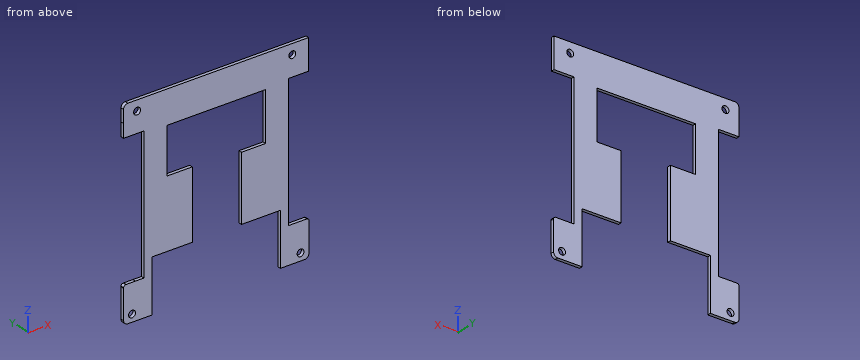
from build123d import *

# Parameters (mm, degrees)
SKETCH1_2_R                 = 1.6383
BOSS_EXTRUDE2_DEPTH         = 1.575
SKETCH2_W                   = 14.080651801
SKETCH2_H                   = 7.11628052
SKETCH2_W_2                 = 15.007196354
SKETCH2_H_2                 = 9.421332762
CUT_EXTRUDE1_DEPTH          = 65.400942629
ADDITIONAL_PCB_MATERIAL_W   = 2.649520344
ADDITIONAL_PCB_MATERIAL_H   = 65.213315835
ADDITIONAL_PCB_MATERIAL_W_2 = 1.5
ADDITIONAL_PCB_MATERIAL_H_2 = 65.299191064
BOSS_EXTRUDE3_DEPTH         = 1.575


with BuildPart() as part:
    # Sketch1_2 → Boss-Extrude2 (new body)
    with BuildSketch(Plane(origin=(0, 0, 0), x_dir=(1, 0, 0), z_dir=(0, 1, 0))):
        with BuildLine():
            Line((-38.39500299, 29.999999735), (-42.73000299, 29.999999735))
            Line((-42.73000299, 29.999999735), (-43.011025994, 30.003097626))
            ThreePointArc((-43.011025994, 30.003097626), (-43.710996344, 30.299838092), (-44.000003042, 31.003036872))
            Line((-44.000003042, 31.003036872), (-44.000003042, 31.269999735))
            Line((-44.000003042, 31.269999735), (-44.000005679, 44.999999735))
            ThreePointArc((-44.000005679, 44.999999735), (-43.414218633, 46.414215608), (-42.000002924, 47.000003051))
            Line((-42.000002924, 47.000003051), (-30.435003, 47.000003051))
            Line((-30.435003, 47.000003051), (-30.435003, 22.255357341))
            Line((-30.435003, 22.255357341), (-11.409003, 22.255357341))
            Line((-11.409003, 22.255357341), (-11.409003, -9.899999999))
            Line((-11.409003, -9.899999999), (-23.409003, -9.899999999))
            Line((-23.409003, -9.899999999), (-23.409003, -31.499996949))
            Line((-23.409003, -31.499996949), (23.408997, -31.499996949))
            Line((23.408997, -31.499996949), (23.408997, -8.499997555))
            Line((23.408997, -8.499997555), (11.97084713, -8.499997555))
            Line((11.97084713, -8.499997555), (11.97084713, 22.255357341))
            Line((11.97084713, 22.255357341), (30.434997, 22.255357341))
            Line((30.434997, 22.255357341), (30.434997, 47.000003051))
            Line((30.434997, 47.000003051), (42.000008541, 47.000003051))
            ThreePointArc((42.000008541, 47.000003051), (43.414213215, 46.414220704), (43.999996956, 45.000016607))
            Line((43.999996956, 45.000016607), (43.999996956, 32.000003378))
            Line((43.999996956, 32.000003378), (43.999996956, 31.015615364))
            ThreePointArc((43.999996956, 31.015615364), (43.706534093, 30.307939396), (42.998386406, 30.015616661))
            Line((42.998386406, 30.015616661), (33.825607551, 30.030389905))
            ThreePointArc((33.825607551, 30.030389905), (33.117459864, 29.738067169), (32.823997, 29.030391202))
            Line((32.823997, 29.030391202), (32.823997, -30.453996949))
            ThreePointArc((32.823997, -30.453996949), (33.116890219, -31.16110373), (33.823997, -31.453996949))
            Line((33.823997, -31.453996949), (36.099999555, -31.453996949))
            Line((36.099999555, -31.453996949), (42.849728118, -31.453996949))
            ThreePointArc((42.849728118, -31.453996949), (43.556834899, -31.746890168), (43.849728118, -32.453996949))
            Line((43.849728118, -32.453996949), (43.849728118, -36.999996949))
            Line((43.849728118, -36.999996949), (43.849728118, -46.999996949))
            Line((43.849728118, -46.999996949), (-42.000000178, -46.999996949))
            ThreePointArc((-42.000000178, -46.999996949), (-43.414212804, -46.414211581), (-44.000000499, -44.999999921))
            Line((-44.000000499, -44.999999921), (-44.000000178, -38.976999921))
            Line((-44.000000178, -38.976999921), (-44.000000178, -32.453999802))
            ThreePointArc((-44.000000178, -32.453999802), (-43.70710696, -31.746893021), (-43.000000178, -31.453999802))
            Line((-43.000000178, -31.453999802), (-36.100000549, -31.453999802))
            Line((-36.100000549, -31.453999802), (-33.824003042, -31.453999802))
            ThreePointArc((-33.824003042, -31.453999802), (-33.116896261, -31.161106583), (-32.824003042, -30.453999802))
            Line((-32.824003042, -30.453999802), (-32.824003042, 29.011483943))
            ThreePointArc((-32.824003042, 29.011483943), (-33.117785331, 29.719478678), (-33.826516131, 30.011480785))
            Line((-33.826516131, 30.011480785), (-38.39500299, 29.999999735))
        make_face()
        with Locations(Location((40, 43.5, 0), (0, 0, 270))):
            Circle(SKETCH1_2_R, mode=Mode.SUBTRACT)
        with Locations(Location((-40, 43.5, 0), (0, 0, 270))):
            Circle(SKETCH1_2_R, mode=Mode.SUBTRACT)
        with Locations(Location((-37.6, -42.2, 0), (0, 0, 270))):
            Circle(SKETCH1_2_R, mode=Mode.SUBTRACT)
        with Locations(Location((36.1, -42.2, 0), (0, 0, 270))):
            Circle(SKETCH1_2_R, mode=Mode.SUBTRACT)
    extrude(amount=BOSS_EXTRUDE2_DEPTH)

    # Sketch2 → Cut-Extrude1 (cut, through all)
    with BuildSketch(Plane(origin=(0, 1.575, 0), x_dir=(1, 0, 0), z_dir=(0, 1, 0))):
        with Locations((39.863054019, -29.135856689)):
            Rectangle(SKETCH2_W, SKETCH2_H)
        with Locations((-40.336598676, -27.983330568)):
            Rectangle(SKETCH2_W_2, SKETCH2_H_2)
    extrude(amount=-CUT_EXTRUDE1_DEPTH, mode=Mode.SUBTRACT)

    # Additional PCB material → Boss-Extrude3 (add)
    with BuildSketch(Plane(origin=(0, 1.575, 0), x_dir=(1, 0, 0), z_dir=(0, 1, 0))):
        with Locations((32.999236828, -1.128517583)):
            Rectangle(ADDITIONAL_PCB_MATERIAL_W, ADDITIONAL_PCB_MATERIAL_H)
        with Locations((-33.574003042, -1.085579968)):
            Rectangle(ADDITIONAL_PCB_MATERIAL_W_2, ADDITIONAL_PCB_MATERIAL_H_2)
    extrude(amount=-BOSS_EXTRUDE3_DEPTH)


solid = part.part
Read the model definition and answer for the solid it produces. Units are mm, in the model's axes. Coordinates: 2 decimals unless noted, no trailing zeros. Order: outer loops, then holes, each group sorted by start corner. A loop starts at its lowest first (then second) coordinate and runs counter-clockwise, first axis right, second up. Notation, with made-up numbers: (57.5, 30.5) - (65.5, 30.5) arc R18 ccw to (65.5, 36.5) - close; hole circle Ø4 at (-7, -1). An arc over 180 degrees is marked (long way). Use one line per item in the form item = value.
(1) Given pin 1 Ø5 at (x, z) = (36.1, 42.2) entering from -Y; pin 2 Ø6 at (x, z) = (10.5, 27.5) entering from -Y (3 decimals); pin 3 Ø0.5 at (y, z) = (0.5, -2) entering from -X; pin 4 Ø0.8 at (y, z) = (1, 25.5) entering from +X, each flat-ended and moving along its own axis, determine where each tip first touches the part or whether it passes through.
Computed values:
pin_1 = 0
pin_2 = through
pin_3 = -34.32
pin_4 = 34.32
(2) Section C-C, the plane z = 42.2 is taken. Give the vertices of the cut face in (x, y) (3 decimals), then the cut area to 3 significant figures.
Computed values:
outline = (-44, 0) - (-39.238, 0) - (-39.238, 1.575) - (-44, 1.575) - close; (-35.962, 0) - (34.462, 0) - (34.462, 1.575) - (-35.962, 1.575) - close; (37.738, 0) - (43.85, 0) - (43.85, 1.575) - (37.738, 1.575) - close
area = 128 mm²
(3) Straight lines are drawn through the part: L1, parallel to X at y = 0.8, z = 42.2; L2, parallel to X at y = 0.5, z = -43.5 (3 decimals); L3, parallel to X at y = 1.3, z = -18.5. For each, find the intervals that lie inside material, in ascending order.
Computed values:
L1 = -44 to -39.24, -35.96 to 34.46, 37.74 to 43.85
L2 = -44 to -41.638, -38.362 to -30.435, 30.435 to 38.362, 41.638 to 44
L3 = -34.32 to -11.41, 11.97 to 34.32
(4) Section A-A, the plane z = -24 is taken. Give the vertices of the cut face in (x, y) (3 decimals), then the cut area to 3 significant figures.
Computed values:
outline = (-34.324, 0) - (-30.435, 0) - (-30.435, 1.575) - (-34.324, 1.575) - close; (30.435, 0) - (34.324, 0) - (34.324, 1.575) - (30.435, 1.575) - close
area = 12.3 mm²
(5) Section B-B, the plane x = -21 is taken. Give the vertices of the cut face in (y, z) (3 decimals), then the cut area to 3 significant figures.
Computed values:
outline = (0, -22.255) - (1.575, -22.255) - (1.575, 9.9) - (0, 9.9) - close; (0, 31.5) - (1.575, 31.5) - (1.575, 47) - (0, 47) - close
area = 75.1 mm²
(6) Section D-D, the plane x = 40 is taken. Give the vertices of the cut face in (y, z) (3 decimals), then the cut area to 3 significant figures.
Computed values:
outline = (0, -47) - (1.575, -47) - (1.575, -45.138) - (0, -45.138) - close; (0, -41.862) - (1.575, -41.862) - (1.575, -30.02) - (0, -30.02) - close; (0, 32.694) - (1.575, 32.694) - (1.575, 47) - (0, 47) - close
area = 44.1 mm²
